Input: part model. Units: mm. Frame: model coordinates. A direction names the side the tool comes from. Coordinates: 2 decimals unless noted, no trailing zeros. Order: outer loops, then holes, each group sorted by start corner. A loop starts at its lowest first (then second) coordinate and runs counter-clockwise, first axis right, second up. Notation, with made-up numbers: (-36, 71.5) -> (15, 71.5) arc R15 cw to (15, 80.5) -> close; hole circle Ø4 at (-38.75, 82.5). An arc over 180 degrees is marked (long way). Answer as CSV lines item,"result".
from build123d import *

# Parameters (mm, degrees)
F0_W     = 50.8
F0_H     = 50.8
F0_W_2   = 38.1
F0_H_2   = 25.4
F1_DEPTH = 25.4


# Not quite as in the source:
# - a feature names something its author has since deleted; it is built from what else it names


with BuildPart() as f1:
    # F0 (on Front) → F1 (new body)
    with BuildSketch(Plane.XZ):
        with Locations((-196.0164945363, -25.4)):
            Rectangle(F0_W, F0_H)
        with Locations((57.9835054637, -25.4)):
            Rectangle(F0_W, F0_H)
        Polygon((32.5835054637, -355.6), (83.3835054637, -355.6), (83.3835054637, -152.4), (57.9835054637, -152.4), (57.9835054637, -133.35), (83.3835054637, -133.35), (83.3835054637, -50.8), (32.5835054637, -50.8), align=None)
        Polygon((-170.6164945363, -355.6), (-170.6164945363, -50.8), (-221.4164945363, -50.8), (-221.4164945363, -133.35), (-196.0164945363, -133.35), (-196.0164945363, -152.4), (-221.4164945363, -152.4), (-221.4164945363, -355.6), align=None)
        Polygon((-170.6164945363, -50.8), (32.5835054637, -50.8), (32.5835054637, 0), (-30.9164945363, 0), (-30.9164945363, -25.4), (-49.9664945363, -25.4), (-88.0664945363, -25.4), (-107.1164945363, -25.4), (-107.1164945363, 0), (-170.6164945363, 0), align=None)
        with Locations((-69.0164945363, -12.7)):
            Rectangle(F0_W_2, F0_H_2)
    extrude(amount=F1_DEPTH)


solid = f1.part
1. Cut plane B-B (y = -6.5). Return the cut outline in (x, z), plus the area to 3 significant figures.
Findings:
outline,"(-221.42, -355.6) -> (-170.62, -355.6) -> (-170.62, -50.8) -> (32.58, -50.8) -> (32.58, -355.6) -> (83.38, -355.6) -> (83.38, -152.4) -> (57.98, -152.4) -> (57.98, -133.35) -> (83.38, -133.35) -> (83.38, 0) -> (-30.92, 0) -> (-30.92, -25.4) -> (-49.97, -25.4) -> (-49.97, 0) -> (-88.07, 0) -> (-88.07, -25.4) -> (-107.12, -25.4) -> (-107.12, 0) -> (-221.42, 0) -> (-221.42, -133.35) -> (-196.02, -133.35) -> (-196.02, -152.4) -> (-221.42, -152.4) -> close"
area,"44,500 mm2"
2. Reachability of faces 1 (the face through (-170.616, -13, -205)), 2 (the face through (57.984, -13, -143)), 3 (the face through (-49.966, -13, -13)), 4 (the face through (-196.016, -13, -143)) from +Z, -Z, +X, -X, +Y, -Y: full face, straight path, thin tool, end or side. Return the list, or none.
Findings:
face 1,"-Z, +Y, -Y"
face 2,"+X, +Y, -Y"
face 3,"+Z, +Y, -Y"
face 4,"-X, +Y, -Y"
3. Cut plane C-C (x = -43.5). Return the cut outline in (y, z).
Findings:
outline,"(-25.4, -50.8) -> (0, -50.8) -> (0, -25.4) -> (-25.4, -25.4) -> close"
4. Cut plane A-A (z = -210). Return the cut outline in (x, y), plus the area to 3 significant figures.
Findings:
outline,"(-221.42, -25.4) -> (-170.62, -25.4) -> (-170.62, 0) -> (-221.42, 0) -> close; (32.58, -25.4) -> (83.38, -25.4) -> (83.38, 0) -> (32.58, 0) -> close"
area,"2,580 mm2"
5. Cut plane D-D (x = 25.5). Return the cut outline in (y, z).
Findings:
outline,"(-25.4, -50.8) -> (0, -50.8) -> (0, 0) -> (-25.4, 0) -> close"
6. Ray query, line 1 along X through (y, z) = (-19.75, -138); line 2 along X through (y, z) = (-16.5, -127); line 3 along Z through (x, y) = (-51.5, -3). Return the intervals inside material, ascending.
Findings:
line 1,"x = -196.02 to -170.62, 32.58 to 57.98"
line 2,"x = -221.42 to -170.62, 32.58 to 83.38"
line 3,"z = -50.8 to 0"
7. Contact query for flat-ended pins moving along their axis: pin 1 (7.5 mm diameter, centred on x = 65.5, y = -14, fed in from +Z); pin 2 (1.5 mm diameter, centred on x = -50, y = -5, fed in from -Z); pin 3 (4 mm diameter, centred on x = -35, y = -15.5, fed in from +Z); pin 4 (9.5 mm diameter, centred on y = -11, z = -145, fed in from +X). Output: stop coordinate, or through.
Findings:
pin 1,"stops at z = 0"
pin 2,"stops at z = -50.8"
pin 3,"stops at z = -25.4"
pin 4,"stops at x = 57.98"
8. Mould query, pull axis Z, two halves, no side actions, for faces 5 (the face through (-209, -13, -133.35)), 6 (the face through (-69, -13, 0)), 7 (the face through (-171, -25.4, -137)). Classes: released by +Z, released by -Z, zero draft, split by the parting line, or undercut.
Findings:
face 5,"undercut"
face 6,"released by +Z"
face 7,"zero draft"
